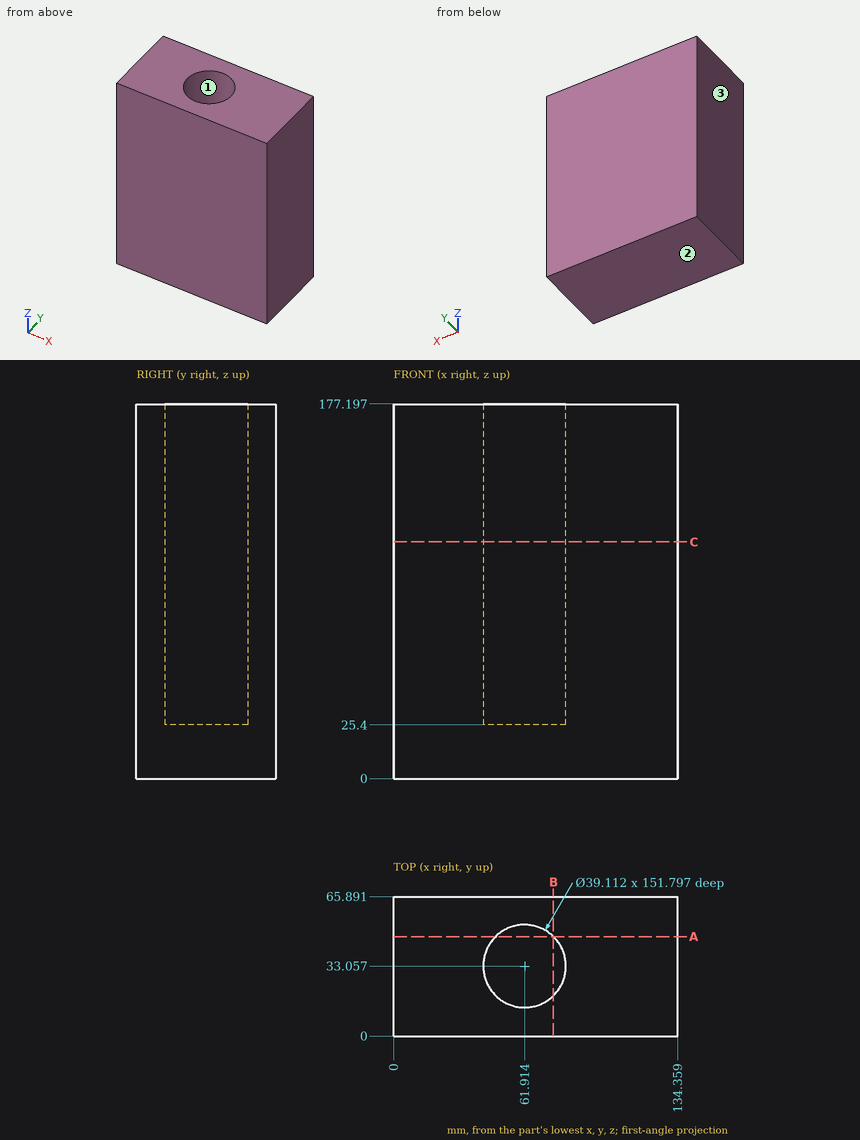
Answer from the drawing. Dimensions are ordinates in mm from the lowest x, y and z of the part. Give positions to 0.01 mm unless a question says otherwise; leave off trailing zeros. Order: outer loops, then holes, each group sorted by start corner. A loop starts at its lowest first (then second) coordinate and runs counter-clockwise, first axis right, second up. Notation, with made-up numbers: (68.5, 40) - (100.5, 40) arc R19 cw to (100.5, 58) - close; hole circle Ø3 at (-2.75, 37). An arc over 180 degrees is marked (long way). One line per item, written item: value. Start each with the question number.
1) Find the intervals of material crossed by L1, parallel to Y at x = 61, z = 119.5; L2, parallel to X at y = 22, z = 162 (1 decimal); L3, parallel to X at y = 38.5, z = 148, in increasing order.
2) A cutting plane is placed at A-A on y = 47. Give the vertices of the cut face in (x, z), then the cut area to 3 significant figures.
3) A cutting plane is placed at C-C on z = 112. Give the vertices of the cut face in (x, y), then the cut area to 3 significant figures.
4) The mould has two halves that part along X. Classify the marked faces 1, 2 and 3: released by +X, released by -X, zero draft, split by the parting line, or undercut.
5) Given pin 1 Ø23.5 at (x, y) = (61.91, 33.06) entering from +Z, flat-ended and moving along its own axis, determine where the tip first touches the part or whether it passes through.
6) A cutting plane is placed at B-B on x = 75.5. Give the vertices of the cut face in (y, z).
Answer sheet:
1. L1: y = 0 to 13.52, 52.59 to 65.89
1. L2: x = 0 to 45.8, 78 to 134.4
1. L3: x = 0 to 43.13, 80.7 to 134.36
2. outline: (0, 0) - (134.36, 0) - (134.36, 177.2) - (75.63, 177.2) - (75.63, 25.4) - (48.2, 25.4) - (48.2, 177.2) - (0, 177.2) - close
2. area: 19,600 mm2
3. outline: (0, 0) - (134.36, 0) - (134.36, 65.89) - (0, 65.89) - close; hole circle Ø39.11 at (61.91, 33.06)
3. area: 7,650 mm2
4. face 1: undercut
4. face 2: zero draft
4. face 3: released by -X
5. pin 1: stops at z = 25.4
6. outline: (0, 0) - (65.89, 0) - (65.89, 177.2) - (47.12, 177.2) - (47.12, 25.4) - (18.99, 25.4) - (18.99, 177.2) - (0, 177.2) - close
